Here's how the part is built. I have some questions about the finished solid (model axes, mm). A direction names the side the tool comes from. Coordinates: 2 decimals unless noted, no trailing zeros. Write each loop counter-clockwise with the first axis right and the second up, starting at its lowest first coordinate (ties: lowest second). Pieces come first, ordered by that corner, then holes.
Item 1: If I drill on line 1 (Z direction, x = 129, y = 0.35); line 2 (Z direction, x = 16.5, y = 0.95); line 3 (Z direction, x = 170.5, y = 0.5), over which ranges is the centre line in solid material (lowest first)?
Item 2: We'd pull the mould along X, two halves only. Please class faces 4 (the face through (165.942, 0.493, -163.764)), 5 (the face through (123, 0, -114)), 6 (the face through (5.2, 0.5, -159.8)), 7 (the face through (88.96, 0.51, -152.36)): +X half, -X half, draft (parallel to the pull), parting line (faces both ways), or undercut.
Item 3: If we section it at C-C (y = 0.5): Count the separate pieces of the cut face and the enclosed holes in it, then the cut area to 3 significant figures.
Item 4: If we section it at A-A (x = 197): Please give me the cut outline in (y, z), then the cut area to 3 significant figures.
Item 5: For faces 1 (the face through (99.297, 0.507, -173.543)), 2 (the face through (4.93, 0.493, -244.636)), 3 (the face through (140.846, 0.507, -74.577)), which set-ups out of +Z, -Z, +X, -X, +Y, -Y let a thin tool reach every point of the face, with its end or its side?
Item 6: If we section it at B-B (z = 3.5): Please give me the cut outline in (x, y), then the cut area to 3 significant figures.
from build123d import *

# Parameters (mm, degrees)
EXTRUDE_1_DEPTH     = 1
SKETCH_2_W          = 80
SKETCH_2_H          = 140
CUT_EXTRUDE_1_DEPTH = 10
CHAMFER_1_SIZE      = 10
SKETCH_3_R          = 1.6
CUT_EXTRUDE_2_DEPTH = 10
SKETCH_4_R          = 2.1
SKETCH_4_R_2        = 1.6
CUT_EXTRUDE_3_DEPTH = 10
SKETCH_5_R          = 3
CUT_EXTRUDE_4_DEPTH = 10
SKETCH_6_R          = 1.6
CUT_EXTRUDE_5_DEPTH = 4
SKETCH_7_R          = 1.6
CUT_EXTRUDE_6_DEPTH = 4
SKETCH_9_R          = 1.1
CUT_EXTRUDE_7_DEPTH = 10


with BuildPart() as part:
    # 草图1 → 凸台-拉伸1 (new body)
    with BuildSketch(Plane(origin=(0, 0, 0), x_dir=(1, 0, 0), z_dir=(0, 1, 0))):
        with BuildLine():
            Line((0, 249.705627485), (0, 155))
            ThreePointArc((0, 155), (109.601551084, 109.601551084), (155, 0))
            ThreePointArc((155, 0), (109.601551084, -109.601551084), (0, -155))
            Line((0, -155), (0, -249.705627485))
            Line((0, -249.705627485), (80, -249.705627485))
            Line((80, -249.705627485), (249.705627485, -80))
            Line((249.705627485, -80), (249.705627485, 0))
            Line((249.705627485, 0), (249.705627485, 80))
            Line((249.705627485, 80), (80, 249.705627485))
            Line((80, 249.705627485), (0, 249.705627485))
        make_face()
    extrude(amount=EXTRUDE_1_DEPTH)

    # 草图2 → 切除-拉伸1 (cut)
    with BuildSketch(Plane(origin=(0, 1, 0), x_dir=(1, 0, 0), z_dir=(0, 1, 0))):
        with Locations((178.293166859, 0)):
            Rectangle(SKETCH_2_W, SKETCH_2_H)
    extrude(amount=-CUT_EXTRUDE_1_DEPTH, mode=Mode.SUBTRACT)

    # 倒角1
    # the kernel refuses this chamfer: 10 mm, written as the material it adds along each edge
    with BuildSketch(Plane(origin=(218.293166859, 1, -70), x_dir=(0, 0, 1), z_dir=(0, -1, 0)), Plane(origin=(218.293166859, 1, 70), x_dir=(-1, 0, 0), z_dir=(0, -1, 0))) as chamfer_1_piece_1:
        Polygon((CHAMFER_1_SIZE, 0), (0, CHAMFER_1_SIZE), (0, 0), align=None)
    extrude(amount=1)
    # the kernel refuses this chamfer: 10 mm, written as the material it takes off along each edge
    with BuildSketch(Plane(origin=(0, -26.617651024, -155), x_dir=(0.9994423420060535, 0, 0.0333916906648138), z_dir=(0, 1, 0))) as chamfer_1_2_piece_1:
        with BuildLine():
            Line((10.351424106, 0), (-CHAMFER_1_SIZE * 0.0333916906648, CHAMFER_1_SIZE * 0.999442342006))
            Line((-CHAMFER_1_SIZE * 0.0333916906648, CHAMFER_1_SIZE * 0.999442342006), (0, 0))
            ThreePointArc((0, 0), (5.321987279, 0.086367968), (10.351424106, 0))
        make_face()
    extrude(amount=54.235302047, mode=Mode.SUBTRACT)
    with BuildSketch(Plane(origin=(0, -25.71682988, -249.705627485), x_dir=(0, 0, 1), z_dir=(0, 1, 0))) as chamfer_1_2_piece_2:
        Polygon((CHAMFER_1_SIZE, 0), (0, CHAMFER_1_SIZE), (0, 0), align=None)
    extrude(amount=52.433659759, mode=Mode.SUBTRACT)
    with BuildSketch(Plane(origin=(80, -25.926703929, -249.705627485), x_dir=(-1, 0, 0), z_dir=(0, 1, 0)), Plane(origin=(249.705627485, -25.926703929, -80), x_dir=(-0.7071067811865482, 0, -0.7071067811865468), z_dir=(0, 1, 0))) as chamfer_1_2_piece_3:
        Polygon((CHAMFER_1_SIZE, 0), (-CHAMFER_1_SIZE * 0.707106781187, CHAMFER_1_SIZE * 0.707106781187), (0, 0), align=None)
    extrude(amount=52.853407858, mode=Mode.SUBTRACT)
    with BuildSketch(Plane(origin=(249.705627485, -25.926703929, 80), x_dir=(-0.7071067811865481, 0, 0.7071067811865468), z_dir=(0, 1, 0)), Plane(origin=(80, -25.926703929, 249.705627485), x_dir=(-1, 0, 0), z_dir=(0, 1, 0))) as chamfer_1_2_piece_4:
        Polygon((CHAMFER_1_SIZE, 0), (-CHAMFER_1_SIZE * 0.707106781187, -CHAMFER_1_SIZE * 0.707106781187), (0, 0), align=None)
    extrude(amount=52.853407858, mode=Mode.SUBTRACT)
    with BuildSketch(Plane(origin=(0, -25.71682988, 249.705627485), x_dir=(0, 0, -1), z_dir=(0, 1, 0))) as chamfer_1_2_piece_5:
        Polygon((CHAMFER_1_SIZE, 0), (0, -CHAMFER_1_SIZE), (0, 0), align=None)
    extrude(amount=52.433659759, mode=Mode.SUBTRACT)
    with BuildSketch(Plane(origin=(0, -26.617651024, 155), x_dir=(0, 0, 1), z_dir=(0, 1, 0))) as chamfer_1_2_piece_6:
        with BuildLine():
            Line((CHAMFER_1_SIZE, 0), (-0.345651552, 10.345651552))
            ThreePointArc((-0.345651552, 10.345651552), (-0.091390348, 5.321903403), (0, 0))
            Line((0, 0), (CHAMFER_1_SIZE, 0))
        make_face()
    extrude(amount=54.235302047, mode=Mode.SUBTRACT)
    with BuildSketch(Plane(origin=(138.293166859, 28.362248577, -70), x_dir=(1, 0, 0), z_dir=(0, -1, 0))) as chamfer_1_2_piece_7:
        with BuildLine():
            Line((CHAMFER_1_SIZE, 0), (-5.105315746, -9.284275337))
            ThreePointArc((-5.105315746, -9.284275337), (-2.557269233, -4.838266251), (0, 0))
            Line((0, 0), (CHAMFER_1_SIZE, 0))
        make_face()
    extrude(amount=55.724497155, mode=Mode.SUBTRACT)
    with BuildSketch(Plane(origin=(138.293166859, 28.362248577, 70), x_dir=(-0.4818437006338934, 0, 0.8762571815166109), z_dir=(0, -1, 0))) as chamfer_1_2_piece_8:
        with BuildLine():
            Line((10.595377171, 0), (-CHAMFER_1_SIZE * 0.481843700634, -CHAMFER_1_SIZE * 0.876257181517))
            Line((-CHAMFER_1_SIZE * 0.481843700634, -CHAMFER_1_SIZE * 0.876257181517), (0, 0))
            ThreePointArc((0, 0), (5.471769619, -0.090462585), (10.595377171, 0))
        make_face()
    extrude(amount=55.724497155, mode=Mode.SUBTRACT)

    # 草图3 → 切除-拉伸2 (cut)
    with BuildSketch(Plane(origin=(0, 1, 0), x_dir=(1, 0, 0), z_dir=(0, 1, 0))):
        with Locations(Location((98.03122292, -221.774909628, 0), (0, 0, 270))):
            Circle(SKETCH_3_R)
        with Locations(Location((108.637824638, -211.16830791, 0), (0, 0, 270))):
            Circle(SKETCH_3_R)
        with Locations(Location((211.16830791, -108.637824638, 0), (0, 0, 270))):
            Circle(SKETCH_3_R)
        with Locations(Location((221.774909628, -98.03122292, 0), (0, 0, 270))):
            Circle(SKETCH_3_R)
        with Locations(Location((244.705627485, -40, 0), (0, 0, 270))):
            Circle(SKETCH_3_R)
        with Locations(Location((244.705627485, 40, 0), (0, 0, 270))):
            Circle(SKETCH_3_R)
        with Locations(Location((221.774909628, 98.03122292, 0), (0, 0, 270))):
            Circle(SKETCH_3_R)
        with Locations(Location((211.16830791, 108.637824638, 0), (0, 0, 270))):
            Circle(SKETCH_3_R)
        with Locations(Location((108.637824638, 211.16830791, 0), (0, 0, 270))):
            Circle(SKETCH_3_R)
        with Locations(Location((98.03122292, 221.774909628, 0), (0, 0, 270))):
            Circle(SKETCH_3_R)
    extrude(amount=-CUT_EXTRUDE_2_DEPTH, mode=Mode.SUBTRACT)

    # 草图4 → 切除-拉伸3 (cut)
    with BuildSketch(Plane(origin=(0, 1, 0), x_dir=(1, 0, 0), z_dir=(0, 1, 0))):
        with Locations(Location((170.793166859, -76.5, 0), (0, 0, 270))):
            Circle(SKETCH_4_R)
        with Locations(Location((185.793166859, -76.5, 0), (0, 0, 270))):
            Circle(SKETCH_4_R)
        with Locations(Location((178.293166859, 91, 0), (0, 0, 270))):
            Circle(SKETCH_4_R_2)
        with Locations(Location((178.293166859, 79.5, 0), (0, 0, 270))):
            Circle(SKETCH_4_R_2)
    extrude(amount=-CUT_EXTRUDE_3_DEPTH, mode=Mode.SUBTRACT)

    # 草图5 → 切除-拉伸4 (cut)
    with BuildSketch(Plane(origin=(0, 1, 0), x_dir=(1, 0, 0), z_dir=(0, 1, 0))):
        with Locations(Location((47.5, -242.75, 0), (0, 0, 270))):
            Circle(SKETCH_5_R)
        with Locations(Location((47.5, 242.75, 0), (0, 0, 270))):
            Circle(SKETCH_5_R)
    extrude(amount=-CUT_EXTRUDE_4_DEPTH, mode=Mode.SUBTRACT)

    # 草图6 → 切除-拉伸5 (cut)
    with BuildSketch(Plane(origin=(0, 1, 0), x_dir=(1, 0, 0), z_dir=(0, 1, 0))):
        with Locations(Location((128.699747468, 107.486544033, 0), (0, 0, 270))):
            Circle(SKETCH_6_R)
        with Locations(Location((114.557611845, 121.628679656, 0), (0, 0, 270))):
            Circle(SKETCH_6_R)
        with Locations(Location((128.699747468, -107.486544033, 0), (0, 0, 270))):
            Circle(SKETCH_6_R)
        with Locations(Location((114.557611845, -121.628679656, 0), (0, 0, 270))):
            Circle(SKETCH_6_R)
    extrude(amount=-CUT_EXTRUDE_5_DEPTH, mode=Mode.SUBTRACT)

    # 草图7 → 切除-拉伸6 (cut)
    with BuildSketch(Plane(origin=(0, 1, 0), x_dir=(1, 0, 0), z_dir=(0, 1, 0))):
        with Locations(Location((218.293166859, 70, 0), (0, 0, 270))):
            Circle(SKETCH_7_R)
        with Locations(Location((218.293166859, -70, 0), (0, 0, 270))):
            Circle(SKETCH_7_R)
    extrude(amount=-CUT_EXTRUDE_6_DEPTH, mode=Mode.SUBTRACT)

    # 草图9 → 切除-拉伸7 (cut)
    with BuildSketch(Plane(origin=(0, 1, 0), x_dir=(1, 0, 0), z_dir=(0, 1, 0))):
        with Locations(Location((188.717667607, 133.916892065, 0), (0, 0, 270))):
            Circle(SKETCH_9_R)
        with Locations(Location((140.987959877, 181.646599796, 0), (0, 0, 270))):
            Circle(SKETCH_9_R)
        with Locations(Location((109.69848481, 133.74011537, 0), (0, 0, 270))):
            Circle(SKETCH_9_R)
        with Locations(Location((140.811183182, 102.627416998, 0), (0, 0, 270))):
            Circle(SKETCH_9_R)
        with BuildLine():
            Line((88.838834765, 163.085046789), (110.0520382, 184.298250225))
            ThreePointArc((110.0520382, 184.298250225), (120.658639918, 184.298250225), (120.658639918, 173.691648507))
            Line((120.658639918, 173.691648507), (99.445436483, 152.478445072))
            ThreePointArc((99.445436483, 152.478445072), (88.838834765, 152.478445072), (88.838834765, 163.085046789))
        make_face()
    extrude(amount=-CUT_EXTRUDE_7_DEPTH, mode=Mode.SUBTRACT)


solid = part.part
Answer list:
1. line 1: z = -200.71 to -109.06, -105.91 to -85.93, 85.93 to 105.91, 109.06 to 200.71
1. line 2: z = -249.71 to -154.12, 154.12 to 249.71
1. line 3: z = -159.21 to -70, 70 to 74.42, 78.58 to 159.21
2. face 4: +X half
2. face 5: draft
2. face 6: -X half
2. face 7: undercut
3. separate pieces: 1
3. enclosed holes: 27
3. area: 47,300 mm2
4. outline: (0, -132.71) - (1, -132.71) - (1, -70) - (0, -70) - close; (0, 70) - (1, 70) - (1, 132.71) - (0, 132.71) - close
4. area: 125 mm2
5. face 1: +Y, -Y
5. face 2: -Z, -X, +Y, -Y
5. face 3: -X, +Y, -Y
6. outline: (218.29, 0) - (249.71, 0) - (249.71, 1) - (218.29, 1) - close
6. area: 31.4 mm2
